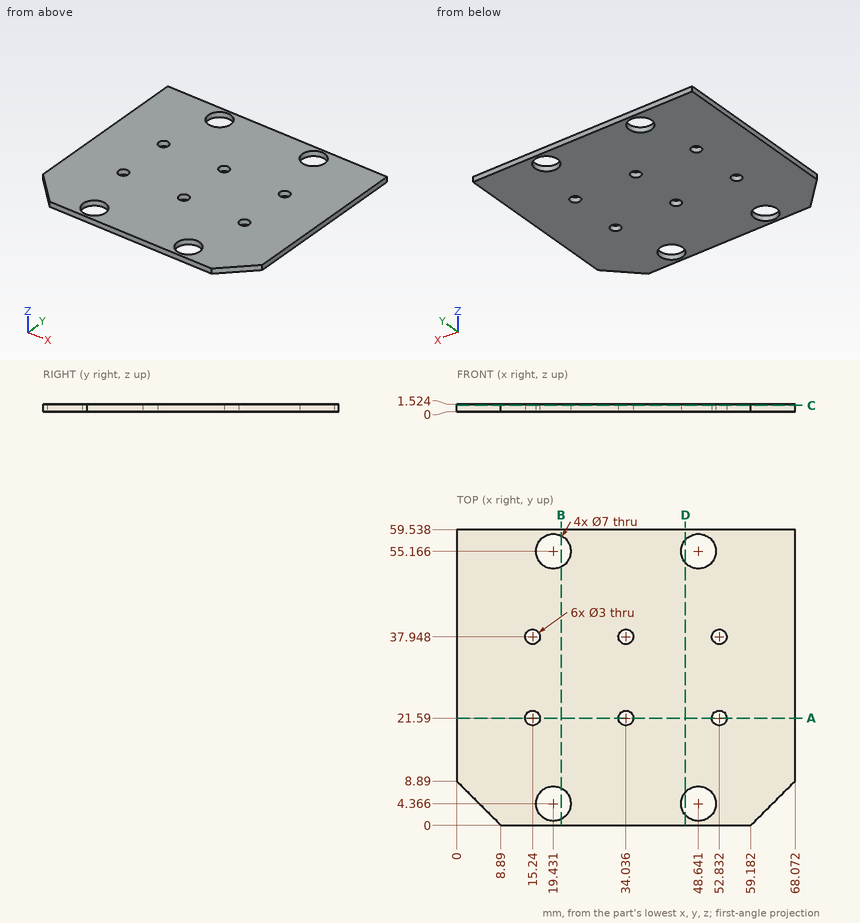
Can you work these out from the drawing? Everything is in mm from the part's minimum corner. Give positions to 0.01 mm unless a question says otherwise; leave off trailing zeros. Order: outer loops, then holes, each group sorted by start corner. A loop starts at its lowest first (then second) coordinate and runs counter-clockwise, first axis right, second up. Notation, with made-up numbers: M 41,86 L 99,86 A12 ccw 99,96 Z; hole C 59,24.25 d1. An arc over 180 degrees is marked long. One line per item, written item: value.
Item 1: If we section it at D-D on x = 46: Write out the boundary of the cut face in (y, z).
Verdict:
outline: M 0,0 L 2.07,0 L 2.07,1.52 L 0,1.52 Z; M 6.66,0 L 52.87,0 L 52.87,1.52 L 6.66,1.52 Z; M 57.46,0 L 59.54,0 L 59.54,1.52 L 57.46,1.52 Z
Item 2: If we section it at A-A on y = 21.59: Write out the boundary of the cut face in (x, z).
Verdict:
outline: M 0,0 L 13.74,0 L 13.74,1.52 L 0,1.52 Z; M 16.74,0 L 32.54,0 L 32.54,1.52 L 16.74,1.52 Z; M 35.54,0 L 51.33,0 L 51.33,1.52 L 35.54,1.52 Z; M 54.33,0 L 68.07,0 L 68.07,1.52 L 54.33,1.52 Z
Item 3: Please list where these lines run through material, in increasing order: line 1 (Y direction, x = 49, z = 0.65) (1 decimal); line 2 (Y direction, x = 15, z = 0.65); line 3 (X direction, y = 3.5, z = 1.3).
Verdict:
line 1: 0 to 0.9, 7.8 to 51.7, 58.6 to 59.5
line 2: 0 to 20.11, 23.07 to 36.47, 39.43 to 59.54
line 3: 5.39 to 16.04, 22.82 to 45.25, 52.03 to 62.68
Item 4: For pin 1 (5.5 mm diameter, centred on x = 19.43, y = 4.37, fed in from +Z), with a flat end and sliding along its axis, tell me the tip position at first contact or that it passes through.
Verdict:
pin 1: through
Item 5: If we section it at C-C on z = 1.25: State how many separate pieces and enclosed holes the cut face has, and give its area (3 significant figures).
Verdict:
separate pieces: 1
enclosed holes: 10
area: 3,780 mm2
Item 6: If we section it at B-B on x = 21: Write out the boundary of the cut face in (y, z) (1 decimal).
Verdict:
outline: M 0,0 L 1.2,0 L 1.2,1.5 L 0,1.5 Z; M 7.5,0 L 52,0 L 52,1.5 L 7.5,1.5 Z; M 58.3,0 L 59.5,0 L 59.5,1.5 L 58.3,1.5 Z
